Autodesk Inventor part; units mm, degrees
ref_plane "YZ Plane" through (0, 0, 0) normal (1, 0, 0) x (0, 1, 0)
ref_plane "XZ Plane" through (0, 0, 0) normal (0, 1, 0) x (-1, 0, 0)
ref_plane "XY Plane" through (0, 0, 0) normal (0, 0, 1) x (1, 0, 0)
sketch "Sketch1" plane through (0, 0, 0) normal (0, 0, 1) x (1, 0, 0)
  line L0 (0, 0) -> (0, 88.9)
  line L1 (12.7, 101.6) -> (38.1, 101.6)
  line L2 (50.8, 88.9) -> (50.8, 50.8)
  arc A0 (12.7, 101.6) -> (0, 88.9) centre (12.7, 88.9) ccw
  arc A1 (50.8, 88.9) -> (38.1, 101.6) centre (38.1, 88.9) ccw
  point P0 (0, 101.6)
  point P1 (50.8, 101.6)
  dimension "d0" = 101.6
  dimension "d1" = 50.8
  dimension "d2" = 50.8
  dimension "d3" = 12.7
sketch "Sketch2" plane through (0, 0, 0) normal (0, 1, 0) x (-1, 0, 0)
  circle A0 centre (0, 0) radius 6.35
  dimension "d4" = 12.7
sweep "Sweep1" add profiles "Sketch2" path "Sketch1"
properties part number "SimpleHook"
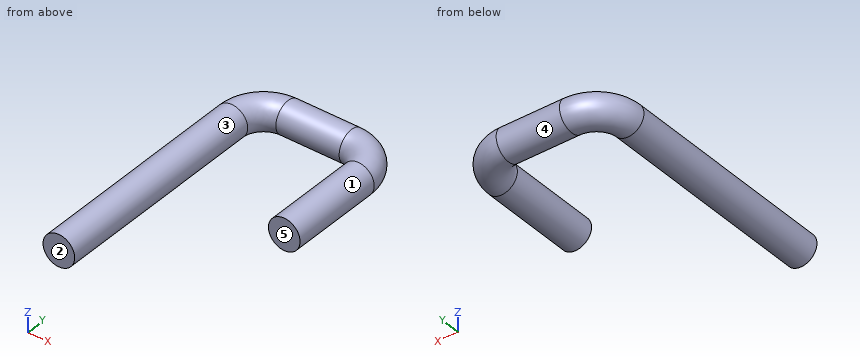
CAD build for the part. Positions are in the model's coordinates, mm. Face numbers are marked on the shaded views. A direction names the side the tool comes from. Coordinates: 2 decimals unless noted, no trailing zeros. Write each loop counter-clockwise with the first axis right and the second up, starting at its lowest first coordinate (ties: lowest second). Pieces come first, ordered by that corner, then holes. Notation, with made-up numbers: (-2, -16) -> (57, -16) arc R27 ccw to (57, 13) -> close; hole circle Ø8 at (-0.75, 71.25). An arc over 180 degrees is marked (long way). Return JSON: item names as keys, results as strings. Group by question number.
Q1. Pull direction X, two halves, no side cores. Call the marked faces 1, 2 and 3: released by +X, released by -X, zero draft, split by the parting line, or undercut.
Q2. Which spindle directions (+Z, -Z, +X, -X, +Y, -Y) get a long thin tool onto all of the face, cutting with end or side? Do the marked faces 4 and 5. Say none if no direction does.
Q3. Flat gauge pins, fed straight in: pin 1 (6 mm diameter, centred on y = 96, z = -1, fed in from +X); pin 2 (3 mm diameter, centred on x = 30.5, y = 95.5, fed in from -Z); pin 3 (6 mm diameter, centred on x = 40.5, z = -4.5, fed in from -Y); pin 4 (6 mm diameter, centred on x = 3, y = 13, fed in from +Z). Where does each tip first touch, or does it go through?
Q4. Cut at B-B, the plane y = 72.5. Give the cut face in (x, z), then the cut area to 3 significant figures.
Q5. Cut at A-A, the plane z = 0. Give the cut face in (x, y), then the cut area to 3 significant figures.
Q6. Cut at D-D, the plane x = 17. Give the cut face in (y, z), then the cut area to 3 significant figures.
Q7. Drill centre lines: line 1 (X direction, y = 24, z = 0.25); line 2 (X direction, y = 89, z = -3.25) (3 decimals). Where is each one in solid material? Low to high.
Q8. Cut at C-C, the plane y = 37. Give the cut face in (x, z), then the cut area to 3 significant figures.
Returned:
{
 "1": {"face 1": "undercut", "face 2": "zero draft", "face 3": "undercut"},
 "2": {"face 4": "none", "face 5": "+Z, -Z, +X, -Y"},
 "3": {"pin 1": "stops at x = 56.68", "pin 2": "stops at z = -4.38", "pin 3": "stops at y = 93.93", "pin 4": "stops at z = 6.35"},
 "4": {"outline": "circle Ø12.7 at (0, 0); circle Ø12.7 at (50.8, 0)", "area": "253 mm2"},
 "5": {"outline": "(-6.35, 0) -> (6.35, 0) -> (6.35, 88.9) arc R6.35 cw to (12.7, 95.25) -> (38.1, 95.25) arc R6.35 cw to (44.45, 88.9) -> (44.45, 50.8) -> (57.15, 50.8) -> (57.15, 88.9) arc R19.05 ccw to (38.1, 107.95) -> (12.7, 107.95) arc R19.05 ccw to (-6.35, 88.9) -> close", "area": "2,440 mm2"},
 "6": {"outline": "circle Ø12.7 at (101.6, 0)", "area": "127 mm2"},
 "7": {"line 1": "x = -6.35 to 6.35", "line 2": "x = -5.455 to 5.456, 45.344 to 56.255"},
 "8": {"outline": "circle Ø12.7 at (0, 0)", "area": "127 mm2"}
}
